Design review of the part built by this model. Coordinates are the model's own, in mm. Coordinates: 2 decimals unless noted, no trailing zeros. Write each loop counter-clockwise with the first axis right and the second up, starting at its lowest first coordinate (ties: lowest second). Pieces come first, ordered by that corner, then holes. Notation, with made-up numbers: (39.25, 80) -> (88.25, 80) arc R29 cw to (88.25, 119) -> close; hole circle Ø3 at (80.5, 30). An arc over 180 degrees is marked (long way). Answer in a Markdown table with one row per item. Add a question column.
Item 1: Take a section at A-A, the plane y = 2. Write out the cut boundary in (x, z).
Item 2: Take a section at D-D, the plane y = -2.5. Write out the cut boundary in (x, z), and give its area (3 significant figures).
Item 3: To check wall thickness, follow line 1 (X direction, y = 8.5, z = 1.5); line 2 (Y direction, x = -64.5, z = 1.2); line 3 (X direction, y = 3.5, z = 3.55). State the ranges of each line that lie inside material, in increasing order.
Item 4: Take a section at C-C, the plane y = -10. Write out the cut boundary in (x, z), and give its area (3 significant figures).
Item 5: Take a section at B-B, the plane x = -64.5. Write out the cut boundary in (y, z).
Item 6: Clearance check with flat-ended pins moving along their axes: P1, Ø0.9, axis at x = -17, z = 2.5, coming from the -Y side; P2, Ø2.5, axis at x = 8, z = 1.5, coming from the -Y side; P3, Ø1.8, axis at x = -64.5, y = -10, coming from the +Z side; P4, Ø2.5, axis at y = -3, z = 3, coming from the +X side. State where each tip first meets the part, or that it passes through.
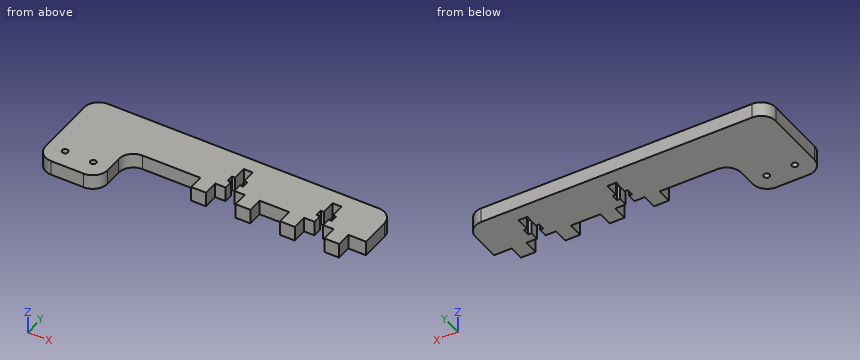
from build123d import *

# Parameters (mm, degrees)
ESQUISSE1_R        = 1
BOSS_EXTRU_1_DEPTH = 5
CONG_1_R           = 5


with BuildPart() as part:
    # Esquisse1 → Boss.-Extru.1 (new body)
    with BuildSketch(Plane.XY):
        Polygon((-16.5, 0), (-20, 0), (-20, -5), (-25, -5), (-25, 0), (-49.542451618, 0), (-49.542451618, -16), (-70.5, -16), (-70.5, 0), (-70.5, 15), (31.001104841, 15), (31.001104841, 0), (25, 0), (25, -5), (20, -5), (20, 0), (16.5, 0), (16.5, 3), (17.6, 3), (17.6, 5.3), (16.5, 5.3), (16.5, 10), (13.5, 10), (13.5, 5.3), (12.4, 5.3), (12.4, 3), (13.5, 3), (13.5, 0), (10, 0), (10, -5), (5, -5), (5, 0), (-5, 0), (-5, -5), (-10, -5), (-10, 0), (-13.5, 0), (-13.5, 3), (-12.4, 3), (-12.4, 5.3), (-13.5, 5.3), (-13.5, 10), (-16.5, 10), (-16.5, 5.3), (-17.6, 5.3), (-17.6, 3), (-16.5, 3), align=None)
        with Locations((-64.5, -10)):
            Circle(ESQUISSE1_R, mode=Mode.SUBTRACT)
        with Locations((-55, -10)):
            Circle(ESQUISSE1_R, mode=Mode.SUBTRACT)
    extrude(amount=BOSS_EXTRU_1_DEPTH)

    # Congé1
    cong_1_edges = [part.edges().sort_by_distance(p)[0] for p in [
        (-49.542451618, 0, 2.5),
        (-49.542451618, -16, 2.5),
        (-70.5, -16, 2.5),
        (-70.5, 15, 2.5),
        (31.001104841, 15, 2.5),
    ]]
    fillet(cong_1_edges, radius=CONG_1_R)


solid = part.part
Answers:
| question | item | result |
|---|---|---|
| 1 | outline | (-70.5, 0) -> (-16.5, 0) -> (-16.5, 5) -> (-70.5, 5) -> close; (-13.5, 0) -> (13.5, 0) -> (13.5, 5) -> (-13.5, 5) -> close; (16.5, 0) -> (31, 0) -> (31, 5) -> (16.5, 5) -> close |
| 2 | outline | (-70.5, 0) -> (-48.87, 0) -> (-48.87, 5) -> (-70.5, 5) -> close; (-25, 0) -> (-20, 0) -> (-20, 5) -> (-25, 5) -> close; (-10, 0) -> (-5, 0) -> (-5, 5) -> (-10, 5) -> close; (5, 0) -> (10, 0) -> (10, 5) -> (5, 5) -> close; (20, 0) -> (25, 0) -> (25, 5) -> (20, 5) -> close |
| 2 | area | 208 mm^2 |
| 3 | line 1 | x = -70.5 to -16.5, -13.5 to 13.5, 16.5 to 31 |
| 3 | line 2 | y = -16 to -11, -9 to 15 |
| 3 | line 3 | x = -70.5 to -17.6, -12.4 to 12.4, 17.6 to 31 |
| 4 | outline | (-70.5, 0) -> (-65.5, 0) -> (-65.5, 5) -> (-70.5, 5) -> close; (-63.5, 0) -> (-56, 0) -> (-56, 5) -> (-63.5, 5) -> close; (-54, 0) -> (-49.54, 0) -> (-49.54, 5) -> (-54, 5) -> close |
| 4 | area | 84.8 mm^2 |
| 5 | outline | (-16, 0) -> (-11, 0) -> (-11, 5) -> (-16, 5) -> close; (-9, 0) -> (15, 0) -> (15, 5) -> (-9, 5) -> close |
| 6 | P1 | stops at y = 0 |
| 6 | P2 | stops at y = -5 |
| 6 | P3 | passes through |
| 6 | P4 | stops at x = 25 |
